from build123d import *

# Parameters (mm, degrees)
SKETCH1_W           = 25
SKETCH1_H           = 80
BOSS_EXTRUDE1_DEPTH = 10
SKETCH2_W           = 25
SKETCH2_H           = 13
BOSS_EXTRUDE2_DEPTH = 86
CUT_EXTRUDE1_DEPTH  = 91
SKETCH4_W           = 20
SKETCH4_H           = 67
CUT_EXTRUDE2_DEPTH  = 5


with BuildPart() as part:
    # Sketch1 → Boss-Extrude1 (new body)
    with BuildSketch(Plane(origin=(0, 0, 0), x_dir=(1, 0, 0), z_dir=(0, 1, 0))):
        Rectangle(SKETCH1_W, SKETCH1_H)
    extrude(amount=BOSS_EXTRUDE1_DEPTH)

    # Sketch2 → Boss-Extrude2 (add)
    with BuildSketch(Plane(origin=(0, 10, 0), x_dir=(1, 0, 0), z_dir=(0, 1, 0))):
        with Locations((0, -33.5)):
            Rectangle(SKETCH2_W, SKETCH2_H)
    extrude(amount=BOSS_EXTRUDE2_DEPTH)

    # Sketch3 → Cut-Extrude1 (cut)
    with BuildSketch(Plane(origin=(0, 96, 0), x_dir=(1, 0, 0), z_dir=(0, 1, 0))):
        Polygon((-4, -27), (4, -27), (4, -31), (7, -31), (4, -35), (-4, -35), (-7, -31), (-4, -31), align=None)
    extrude(amount=-CUT_EXTRUDE1_DEPTH, mode=Mode.SUBTRACT)

    # Sketch4 → Cut-Extrude2 (cut)
    with BuildSketch(Plane(origin=(0, 10, 0), x_dir=(1, 0, 0), z_dir=(0, 1, 0))):
        with Locations((0, 6.5)):
            Rectangle(SKETCH4_W, SKETCH4_H)
    extrude(amount=-CUT_EXTRUDE2_DEPTH, mode=Mode.SUBTRACT)


solid = part.part
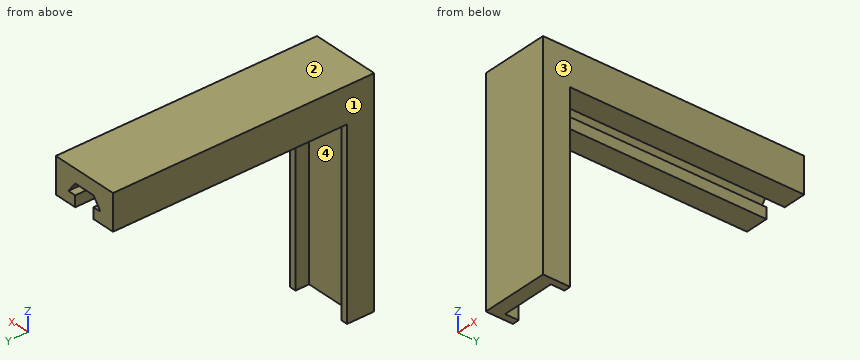
Here's how the part is built. I have some questions about the finished solid (model axes, mm). Face numbers are marked on the shaded views. Round coordinates to 2 decimals unless told otherwise and drop trailing zeros. Write each loop counter-clockwise with the first axis right and the second up, starting at its lowest first coordinate (ties: lowest second). Pieces come first, ordered by that corner, then holes.
1. Suppose I cut it at C-C (y = 7.5). List the corners of the cut face in (x, z) for me, and give its area (3 significant figures).
2. If we mould it in two halves opening along X, with no side actions, what happens to the marked faces 1, 2, 3 and 4? For each: released by +X, released by -X, zero draft, split by the parting line, or undercut.
3. I need wall thicknesses on L1, parallel to X at y = 13, z = 28.5; L2, parallel to Y at x = -4.75, z = -19; L3, parallel to Z at x = 4.75, y = 73. Which ranges of each line are inside material? Lowest first, please.
4. Suppose I cut it at A-A (y = 54.5). List the corners of the cut face in (x, z) for me, and give its area (3 significant figures).
5. Will these pins go through, and if not, where does the flat tip stop? pin 1 Ø9.5 at (x, y) = (-6.5, 37) entering from -Z; pin 2 Ø1.2 at (x, z) = (-11.5, 1.5) entering from +Y; pin 3 Ø10 at (y, z) = (17, 16.5) entering from +X; pin 4 Ø6.5 at (x, y) = (0, 72) entering from -Z.
6. Suppose I cut it at B-B (z = -27). List the corners of the cut face in (x, y) for me.
Answer sheet:
1. outline: (-12.5, -40) - (-10, -40) - (-10, 27) - (-4, 27) - (-4, 31) - (-7, 31) - (-4, 35) - (4, 35) - (7, 31) - (4, 31) - (4, 27) - (10, 27) - (10, -40) - (12.5, -40) - (12.5, 40) - (-12.5, 40) - close
1. area: 584 mm2
2. face 1: released by -X
2. face 2: zero draft
2. face 3: released by +X
2. face 4: undercut
3. L1: x = -12.5 to -4, 4 to 12.5
3. L2: y = 0 to 5
3. L3: z = 27 to 31, 34 to 40
4. outline: (-12.5, 27) - (-4, 27) - (-4, 31) - (-7, 31) - (-4, 35) - (4, 35) - (7, 31) - (4, 31) - (4, 27) - (12.5, 27) - (12.5, 40) - (-12.5, 40) - close
4. area: 249 mm2
5. pin 1: stops at z = 27
5. pin 2: stops at y = 10
5. pin 3: passes through
5. pin 4: stops at z = 35
6. outline: (-12.5, 0) - (12.5, 0) - (12.5, 10) - (10, 10) - (10, 5) - (-10, 5) - (-10, 10) - (-12.5, 10) - close
